from build123d import *

# Parameters (mm, degrees)
F0_R     = 63.5
F1_DEPTH = 6.35
F3_DEPTH = 6.35
F4_W     = 12.7
F4_H     = 12.7
F5_DEPTH = 6.35
F6_R     = 10.15999
F7_R     = 5.08
F8_W     = 8.89
F8_H     = 19.05
F9_DEPTH = 6.35


# Not quite as in the source:
# - a fillet or chamfer is up to 0.001 mm smaller than in the source, because OpenCascade refuses the exact size
# - a feature names something its author has since deleted; it is built from what else it names


with BuildPart() as f1:
    # F0 (on Top) → F1 (new body)
    with BuildSketch(Plane.XY):
        Circle(F0_R)
    extrude(amount=F1_DEPTH)

    # F2 (on face) → F3 (join)
    with BuildSketch(Plane.XY.offset(6.35)):
        Polygon((-21.59, 0), (-25.4, 0), (-29.21, 0), (-35.56, -6.35), (-35.56, -38.1), (-15.24, -38.1), (-15.24, -6.35), align=None)
        Polygon((-29.21, 0), (-25.4, 0), (-21.59, 0), (-15.24, 6.35), (-15.24, 38.1), (-35.56, 38.1), (-35.56, 6.35), align=None)
    extrude(amount=F3_DEPTH)

    # F4 (on face) → F5 (join)
    with BuildSketch(Plane.XY.offset(6.35)):
        Polygon((12.7, 38.1), (12.7, 0), (12.7, -38.1), (25.4, -38.1), (25.4, -25.4), (25.4, -6.35), (25.4, 0), (25.4, 6.35), (25.4, 25.4), (25.4, 38.1), align=None)
        with Locations((31.75, 31.75)):
            Rectangle(F4_W, F4_H)
        with Locations((31.75, -31.75)):
            Rectangle(F4_W, F4_H)
        Polygon((38.1, 6.35), (25.4, 6.35), (25.4, 0), (25.4, -6.35), (38.1, -6.35), align=None)
    extrude(amount=F5_DEPTH)

    # F6 (radius 10.16 in the source; OpenCascade refuses exactly that, so slightly less here)
    f6_edges = [f1.edges().sort_by_distance(p)[0] for p in [
        (-35.56, -38.1, 9.525),
        (-15.24, -38.1, 9.525),
        (-15.24, 38.1, 9.525),
        (-35.56, 38.1, 9.525),
    ]]
    fillet(f6_edges, radius=F6_R)

    # F7
    f7_edges = [f1.edges().sort_by_distance(p)[0] for p in [
        (38.1, 6.35, 9.525),
        (38.1, -6.35, 9.525),
        (38.1, -38.1, 9.525),
        (38.1, -25.4, 9.525),
        (38.1, 25.4, 9.525),
        (38.1, 38.1, 9.525),
        (12.7, 38.1, 9.525),
        (12.7, -38.1, 9.525),
    ]]
    fillet(f7_edges, radius=F7_R)

    # F8 (on face) → F9 (cut)
    with BuildSketch(Plane.XY.offset(12.7)):
        Polygon((-29.845, -28.575), (-20.955, -28.575), (-20.955, -9.525), (-25.4, -9.525), (-29.845, -9.525), align=None)
        with Locations((-25.4, 19.05)):
            Rectangle(F8_W, F8_H)
    extrude(amount=-F9_DEPTH, mode=Mode.SUBTRACT)


solid = f1.part
Could you check a few things on this model? Use its own coordinates, in mm. A direction names the side the tool comes from. Give positions to 0.01 mm unless a question says otherwise; leave off trailing zeros. Loops run counter-clockwise (first coordinate to the right, second up) from the corner with the lowest first, then second, coordinate; pieces in that order, holes last. Notation, with made-up numbers: (-5.5, 31) -> (18.5, 31) arc R10 ccw to (18.5, 50) -> close; hole circle Ø4 at (33.5, -33). An arc over 180 degrees is marked (long way). Answer as CSV lines item,"result". Start each with the question number.
(1) If we section it at C-C on y = 17: Write out the boundary of the cut face in (x, z) (3 decimals), then the cut area to 3 significant figures.
(2) Which directions (+Z, -Z, +X, -X, +Y, -Y) give clear straight access to the entire face, cutting with the end or side of a thin tool? Please do faces 4 (the cylindrical face through (-32.663, 35.045, 9.569)), 5 (the flat face through (-35.56, 17, 9)), 6 (the flat face through (-20.955, -19, 10)), 7 (the flat face through (29, -25.4, 9)), 8 (the cylindrical face through (-18.295, 35.203, 9.569)).
(3) I'm going to push flat-ended pins straight in: pin 1 Ø5 at (x, z) = (25.5, 6.5) entering from +Y; pin 2 Ø4.5 at (x, y) = (-25, 18) entering from +Z; pin 3 Ø7 at (y, z) = (-16.5, 9.5) entering from +X. Where does each tip first touch, or does it pass through?
(4) If we section it at A-A on x = 20: Write out the boundary of the cut face in (y, z), then the cut area to 3 significant figures.
(5) If we section it at D-D on y = -19: Write out the boundary of the cut face in (x, z) (3 decimals), then the cut area to 3 significant figures.
(6) I need wall thicknesses on probe 1 along Y at (x, z) = (-25.5, 9) (1 decimal); probe 2 along X at (y, z) = (23.5, 10.5) (3 decimals); probe 3 along Z at (x, y) = (47.5, 14.5). Which ranges of each line are inside material? Lowest first, please.
(7) We'd pull the mould along Y, two halves only. Please class faces 1 (the flat face through (26, 38.1, 9)), 2 (the cylindrical face through (36.651, -26.928, 9.569)), 3 (the flat face through (-15.24, 17, 9)): released by +Y, released by -Y, zero draft, split by the parting line, or undercut.
(8) If we section it at B-B on z = 2.75: Write out the boundary of the cut face in (x, y).
Computed:
1,outline,"(-61.182, 0) -> (61.182, 0) -> (61.182, 6.35) -> (25.4, 6.35) -> (25.4, 12.7) -> (12.7, 12.7) -> (12.7, 6.35) -> (-15.24, 6.35) -> (-15.24, 12.7) -> (-20.955, 12.7) -> (-20.955, 6.35) -> (-29.845, 6.35) -> (-29.845, 12.7) -> (-35.56, 12.7) -> (-35.56, 6.35) -> (-61.182, 6.35) -> close"
1,area,"930 mm2"
2,face 4,"+Z, -X, +Y"
2,face 5,"+Z, -X, +Y, -Y"
2,face 6,"+Z"
2,face 7,"+Z, +X"
2,face 8,"+Z, +Y"
3,pin 1,"stops at y = 59.19"
3,pin 2,"stops at z = 6.35"
3,pin 3,"stops at x = 61.71"
4,outline,"(-60.27, 0) -> (60.27, 0) -> (60.27, 6.35) -> (38.1, 6.35) -> (38.1, 12.7) -> (-38.1, 12.7) -> (-38.1, 6.35) -> (-60.27, 6.35) -> close"
4,area,"1,250 mm2"
5,outline,"(-60.591, 0) -> (60.591, 0) -> (60.591, 6.35) -> (25.4, 6.35) -> (25.4, 12.7) -> (12.7, 12.7) -> (12.7, 6.35) -> (-15.24, 6.35) -> (-15.24, 12.7) -> (-20.955, 12.7) -> (-20.955, 6.35) -> (-29.845, 6.35) -> (-29.845, 12.7) -> (-35.56, 12.7) -> (-35.56, 6.35) -> (-60.591, 6.35) -> close"
5,area,"923 mm2"
6,probe 1,"y = -38.1 to -28.6, -9.5 to 9.5, 28.6 to 38.1"
6,probe 2,"x = -35.56 to -29.845, -20.955 to -15.24, 12.7 to 25.4"
6,probe 3,"z = 0 to 6.35"
7,face 1,"released by +Y"
7,face 2,"undercut"
7,face 3,"zero draft"
8,outline,"circle Ø127 at (0, 0)"
